from build123d import *

# Parameters (mm, degrees)
SKETCH1_W                      = 10
SKETCH1_H                      = 20
SKETCH1_R                      = 1.175
BOSS_EXTRUDE1_DEPTH            = 3
CBORE_FOR_M2_SHCS1_D           = 2.4
CBORE_FOR_M2_SHCS1_CBORE_D     = 4.4
CBORE_FOR_M2_SHCS1_CBORE_DEPTH = 2
SKETCH6_W                      = 10
SKETCH6_H                      = 3
BOSS_EXTRUDE2_DEPTH            = 30
SKETCH8_W                      = 3
SKETCH8_H                      = 25
BOSS_EXTRUDE3_DEPTH            = 15
SKETCH9_R                      = 1.75
CUT_EXTRUDE1_DEPTH             = 36.67912555
FILLET1_R                      = 1
FILLET2_R                      = 1


with BuildPart() as part:
    # Sketch1 → Boss-Extrude1 (new body)
    with BuildSketch(Plane(origin=(0, 0, 0), x_dir=(1, 0, 0), z_dir=(0, 1, 0))):
        with Locations((5, 10)):
            Rectangle(SKETCH1_W, SKETCH1_H)
        with Locations(Location((6.5, 5.25, 0), (0, 0, 270))):
            Circle(SKETCH1_R, mode=Mode.SUBTRACT)
        with Locations(Location((6.5, 14.75, 0), (0, 0, 270))):
            Circle(SKETCH1_R, mode=Mode.SUBTRACT)
    extrude(amount=BOSS_EXTRUDE1_DEPTH)

    # CBORE for M2 SHCS1 (through all)
    with Locations(Plane(origin=(0, 3, 0), x_dir=(1, 0, 0), z_dir=(0, 1, 0))):
        with Locations((6.5, 14.75), (6.5, 5.25)):
            CounterBoreHole(CBORE_FOR_M2_SHCS1_D / 2, CBORE_FOR_M2_SHCS1_CBORE_D / 2, CBORE_FOR_M2_SHCS1_CBORE_DEPTH)

    # Sketch6 → Boss-Extrude2 (add)
    with BuildSketch(Plane(origin=(0, 0, 0), x_dir=(-1, 0, 0), z_dir=(0, 0, -1))):
        with Locations((-5, 1.5)):
            Rectangle(SKETCH6_W, SKETCH6_H)
    extrude(amount=-BOSS_EXTRUDE2_DEPTH)

    # Sketch8 → Boss-Extrude3 (add)
    with BuildSketch(Plane(origin=(0, 3, 0), x_dir=(1, 0, 0), z_dir=(0, 1, 0))):
        with Locations((1.5, -17.5)):
            Rectangle(SKETCH8_W, SKETCH8_H)
    extrude(amount=BOSS_EXTRUDE3_DEPTH)

    # Sketch9 → Cut-Extrude1 (cut, through all)
    with BuildSketch(Plane(origin=(3, 0, 0), x_dir=(0, 0, -1), z_dir=(1, 0, 0))):
        with Locations((-20, 13)):
            Circle(SKETCH9_R)
    extrude(amount=-CUT_EXTRUDE1_DEPTH, mode=Mode.SUBTRACT)

    # Fillet1
    fillet1_edges = [part.edges().sort_by_distance(p)[0] for p in [
        (3, 3, 17.5),
        (1.5, 3, 5),
    ]]
    fillet(fillet1_edges, radius=FILLET1_R)

    # Fillet2
    fillet2_edges = [part.edges().sort_by_distance(p)[0] for p in [
        (0, 0, 5),
    ]]
    fillet(fillet2_edges, radius=FILLET2_R)


solid = part.part
Input: part model. Units: mm. Frame: model coordinates. A direction names the side the tool comes from. Coordinates: 2 decimals unless noted, no trailing zeros. Loops run counter-clockwise (first coordinate to the right, second up) from the corner with the lowest first, then second, coordinate; pieces in that order, holes last. Notation, with made-up numbers: (52.25, -27) -> (110.25, -27) arc R20 ccw to (110.25, -19) -> close; hole circle Ø2 at (5, -0.5). An arc over 180 degrees is marked (long way). One line per item, written item: value.
(1) Cut plane B-B (x = 6.5). Output: boundary loops of the cut face in (y, z), then the cut area to 3 significant figures.
Answer below:
outline: (0, -20) -> (3, -20) -> (3, -16.95) -> (1, -16.95) -> (1, -15.95) -> (0, -15.95) -> close; (0, -13.55) -> (1, -13.55) -> (1, -12.55) -> (3, -12.55) -> (3, -7.45) -> (1, -7.45) -> (1, -6.45) -> (0, -6.45) -> close; (0, -4.05) -> (1, -4.05) -> (1, -3.05) -> (3, -3.05) -> (3, 30) -> (0, 30) -> close
area: 128 mm2
(2) Pin query (flat end, axial travel): pin 1 Ø4 at (x, z) = (6.5, -5.25) entering from -Y; pin 2 Ø7 at (y, z) = (10.5, 11.5) entering from +X; pin 3 Ø1.3 at (x, z) = (6, -14) entering from +Y; pin 4 Ø1.9 at (x, z) = (6.5, -5.25) entering from -Y. Return the tip coordinate at first contact, or that it passes through.
Answer below:
pin 1: stops at y = 0
pin 2: stops at x = 3
pin 3: stops at y = 1
pin 4: passes through
(3) Ray query, line 1 along Z through (x, y) = (6.5, 0.4); line 2 along Z through (x, y) = (7.5, 2); line 3 along Y through (x, z) = (1, 0). Return the intervals inside material, ascending.
Answer below:
line 1: z = -20 to -15.95, -13.55 to -6.45, -4.05 to 30
line 2: z = -20 to -16.71, -12.79 to -7.21, -3.29 to 30
line 3: y = 0 to 3
(4) Cut plane A-A (z = -5.25). Output: boundary loops of the cut face in (x, y).
Answer below:
outline: (0, 1) arc R1 ccw to (1, 0) -> (5.3, 0) -> (5.3, 1) -> (4.3, 1) -> (4.3, 3) -> (0, 3) -> close; (7.7, 0) -> (10, 0) -> (10, 3) -> (8.7, 3) -> (8.7, 1) -> (7.7, 1) -> close
(5) Set-up query: faces 1 (the face through (3, 11, 18)), 2 (the face through (1, 11, 5)), 3 (the face through (8.532, 2.014, -13.907)). Return all of +Z, -Z, +X, -X, +Y, -Y with unobstructed straight access to the full face (end or side cutting, diameter ignored); none if empty.
Answer below:
face 1: +Z, -Z, +X, +Y
face 2: -Z, +X, -X, +Y
face 3: +Y
(6) Cut plane C-C (y = 13). Output: boundary loops of the cut face in (x, z), then the cut area to 3 significant figures.
Answer below:
outline: (0, 5) -> (3, 5) -> (3, 18.25) -> (0, 18.25) -> close; (0, 21.75) -> (3, 21.75) -> (3, 30) -> (0, 30) -> close
area: 64.5 mm2
(7) Cut plane D-D (z = 24). Output: boundary loops of the cut face in (x, y), then the cut area to 3 significant figures.
Answer below:
outline: (0, 1) arc R1 ccw to (1, 0) -> (10, 0) -> (10, 3) -> (4, 3) arc R1 cw to (3, 4) -> (3, 18) -> (0, 18) -> close
area: 75.0 mm2
(8) Draft query along X for faces 4 (the face through (6.76, 0.49, -13.58)), 5 (the face through (6, 3, -1)), 6 (the face through (0, 9, 16)). Return one class per face: pulls with the +X half, pulls with the -X half, needs draft (parallel to the pull), parting line crosses it, or undercut.
Answer below:
face 4: undercut
face 5: needs draft
face 6: pulls with the -X half
